from build123d import *

# Parameters (mm, degrees)
F0_R     = 12
F0_R_2   = 8
F1_DEPTH = 5.15
F2_DEPTH = 5.15
F0_R_3   = 7
F3_DEPTH = 0.22
F4_DEPTH = 0.22
F5_SIZE  = 2


with BuildPart() as f1:
    # F0 (on Front) → F1 (new body)
    with BuildSketch(Plane.XZ):
        Circle(F0_R)
        Circle(F0_R_2, mode=Mode.SUBTRACT)
    extrude(amount=F1_DEPTH)

    # F0 (on Front) → F2 (join)
    with BuildSketch(Plane.XZ):
        Circle(F0_R)
        Circle(F0_R_2, mode=Mode.SUBTRACT)
    extrude(amount=-F2_DEPTH)

    # F0 (on Front) → F3 (join)
    with BuildSketch(Plane.XZ):
        Circle(F0_R_2)
        Circle(F0_R_3, mode=Mode.SUBTRACT)
    extrude(amount=F3_DEPTH)

    # F0 (on Front) → F4 (join)
    with BuildSketch(Plane.XZ):
        Circle(F0_R_2)
        Circle(F0_R_3, mode=Mode.SUBTRACT)
    extrude(amount=-F4_DEPTH)

    # F5
    f5_edges = [f1.edges().sort_by_distance(p)[0] for p in [
        (-12, -5.15, 0),
        (-12, 5.15, 0),
    ]]
    chamfer(f5_edges, length=F5_SIZE)


solid = f1.part
Design review of the part built by this model. Coordinates are the model's own, in mm. A direction names the side the tool comes from. Round coordinates to 2 decimals unless told otherwise and drop trailing zeros. Loops run counter-clockwise (first coordinate to the right, second up) from the corner with the lowest first, then second, coordinate; pieces in that order, holes last. Notation, with made-up numbers: M 74.5,7 L 93.5,7 A15 cw 93.5,28 Z; hole C 6.5,71.25 d4. An arc over 180 degrees is marked long. Answer as a JSON object with one key per item and string values.
Item 1: We need section B-B on x = 0. Give the boundary of the cut face in (y, z), and give its area (3 significant figures).
Answer sheet:
{"outline": "M -5.15,-10 L -3.15,-12 L 3.15,-12 L 5.15,-10 L 5.15,-8 L 0.22,-8 L 0.22,-7 L -0.22,-7 L -0.22,-8 L -5.15,-8 Z; M -5.15,8 L -0.22,8 L -0.22,7 L 0.22,7 L 0.22,8 L 5.15,8 L 5.15,10 L 3.15,12 L -3.15,12 L -5.15,10 Z", "area": "75.3 mm^2"}
Item 2: Clearance check with flat-ended pins moving along their axes: P1, Ø8, axis at x = -2.5, z = 3, coming from the +Y side; P2, Ø3, axis at y = -2, z = -9, coming from the +X side; P3, Ø2, axis at y = 3, z = -1.5, coming from the +X side. State where each tip first meets the part, or that it passes through.
Answer sheet:
{"P1": "stops at y = 0.22", "P2": "stops at x = 9.37", "P3": "stops at x = 11.99"}
Item 3: Machinability: for faces 1 (the cylindrical face through (-1.73, -2.65, -7.81)), 2 (the cylindrical face through (-1.73, 2.65, -7.81)), 3 (the flat face through (0, 5.15, 8.2)), which of the approach directions +Z, -Z, +X, -X, +Y, -Y give a long, thin tool a straight path to every point of the face, cutting with its end or side? Answer none if there is none.
Answer sheet:
{"face 1": "-Y", "face 2": "+Y", "face 3": "+Z, -Z, +X, -X, +Y"}
Item 4: The part is to be moulded in two halves that separate along X. For faces 4 (the flat face through (4, -0.22, -6)), 5 (the flat face through (0, -5.15, 8.2)), 6 (the cylindrical face through (-11.99, -0.04, 0.53)), say which applies: pulls with the +X half, pulls with the -X half, needs draft (parallel to the pull), parting line crosses it, or undercut.
Answer sheet:
{"face 4": "undercut", "face 5": "needs draft", "face 6": "parting line crosses it"}
Item 5: We need section C-C on y = -0.75. Give the boundary of the cut face in (x, z).
Answer sheet:
{"outline": "C 0,0 d24; hole C 0,0 d16"}
Item 6: We need section A-A on z = 0. Give the boundary of the cut face in (x, y), and give its area (3 significant figures).
Answer sheet:
{"outline": "M -12,-3.15 L -10,-5.15 L -8,-5.15 L -8,-0.22 L -7,-0.22 L -7,0.22 L -8,0.22 L -8,5.15 L -10,5.15 L -12,3.15 Z; M 7,-0.22 L 8,-0.22 L 8,-5.15 L 10,-5.15 L 12,-3.15 L 12,3.15 L 10,5.15 L 8,5.15 L 8,0.22 L 7,0.22 Z", "area": "75.3 mm^2"}
Item 7: Wall thickness on L1, parallel to Z at x = 0, y = 1.2; L2, parallel to Z at x = 0, y = -0.05; L3, parallel to X at y = -0.75, z = 1.5: over which ranges is each line inside the solid? List them lowest first. Write a range as from..to.
Answer sheet:
{"L1": "z = -12..-8, 8..12", "L2": "z = -12..-7, 7..12", "L3": "x = -11.91..-7.86, 7.86..11.91"}
